from build123d import *

# Parameters (mm, degrees)
F0_W           = 127
F0_H           = 45.593
F1_DEPTH       = 19.05
F3_D           = 13.5128
F3_DEPTH       = 19.05
F3_CBORE_D     = 20.066
F3_CBORE_DEPTH = 13.4874
F3_TIP         = 4.0596546864
F5_DEPTH       = 45.593
F7_DEPTH       = 10.1854
F9_DEPTH       = 7.9375
F10_R          = 4.7625
F11_DEPTH      = 69.85
F12_R          = 4.76249
F4_R           = 4.7625


# Not quite as in the source:
# - a fillet or chamfer is up to 0.001 mm smaller than in the source, because OpenCascade refuses the exact size


with BuildPart() as f1:
    # F0 (on Front) → F1 (new body)
    with BuildSketch(Plane.XZ):
        with Locations((63.5, -22.7965)):
            Rectangle(F0_W, F0_H)
    extrude(amount=-F1_DEPTH)

    # F3
    with Locations(Plane.XZ):
        with Locations((14.3002, -21.7424), (112.7125, -21.7424)):
            CounterBoreHole(F3_D / 2, F3_CBORE_D / 2, F3_CBORE_DEPTH, depth=F3_DEPTH)
            with Locations((0, 0, -(F3_DEPTH + F3_TIP / 2))):  # 118° drill point
                Cone(0, F3_D / 2, F3_TIP, mode=Mode.SUBTRACT)

    # F4 (on face) → F5 (cut)
    with BuildSketch(Plane.XY):
        with BuildLine():
            Line((58.7375, 0), (68.2625, 0))
            ThreePointArc((68.2625, 0), (63.5, 4.7625), (58.7375, 0))
        make_face()
        with BuildLine():
            ThreePointArc((58.7375, 0), (63.5, -4.7625), (68.2625, 0))
            Line((68.2625, 0), (58.7375, 0))
        make_face()
    extrude(amount=-F5_DEPTH, mode=Mode.SUBTRACT)

    # F6 (on face) → F7 (cut)
    with BuildSketch(Plane.XZ):
        with BuildLine():
            Line((93.6498, 0), (76.2, 0))
            Line((76.2, 0), (76.2, -30.1625))
            ThreePointArc((76.2, -30.1625), (77.1299359697, -32.4075640303), (79.375, -33.3375))
            Line((79.375, -33.3375), (90.4748, -33.3375))
            ThreePointArc((90.4748, -33.3375), (92.7198640303, -32.4075640303), (93.6498, -30.1625))
            Line((93.6498, -30.1625), (93.6498, 0))
        make_face()
    extrude(amount=-F7_DEPTH, mode=Mode.SUBTRACT)

    # F8 (on Front) → F9 (cut)
    with BuildSketch(Plane.XZ):
        with BuildLine():
            Line((103.8733, 0), (95.9358, 0))
            Line((95.9358, 0), (95.9358, -22.1996))
            ThreePointArc((95.9358, -22.1996), (97.0963600902, -25.0014399098), (99.8982, -26.162))
            Line((99.8982, -26.162), (99.9109, -26.162))
            ThreePointArc((99.9109, -26.162), (102.7127399098, -25.0014399098), (103.8733, -22.1996))
            Line((103.8733, -22.1996), (103.8733, 0))
        make_face()
    extrude(amount=-F9_DEPTH, mode=Mode.SUBTRACT)

    # F10 (on face) → F11 (cut)
    with BuildSketch(Plane.YZ.offset(95.9358)):
        with Locations((0, -13.2588)):
            Circle(F10_R)
    extrude(amount=-F11_DEPTH, mode=Mode.SUBTRACT)

    # F12 (radius 4.7625 in the source; OpenCascade refuses exactly that, so slightly less here)
    f12_edges = [f1.edges().sort_by_distance(p)[0] for p in [
        (26.0858, 4.7625, -13.2588),
    ]]
    fillet(f12_edges, radius=F12_R)

    # F14: sweep along a path in F13
    with BuildLine(Plane.XZ) as f14_path:
        Line((63.5, 0), (63.5, -2.4638))
        ThreePointArc((63.5, -2.4638), (66.6617822971, -10.0970177029), (74.295, -13.2588))
        Line((74.295, -13.2588), (77.6987022404, -13.2588))
    # F4 (on face) → F14 (sweep, cut)
    with BuildSketch(Plane.XY):
        with Locations((63.5, 0)):
            Circle(F4_R)
    sweep(path=f14_path.line, mode=Mode.SUBTRACT)


solid = f1.part
Geometry: final body of the model. Coordinates: model frame, mm. A direction names the side the tool comes from. Give positions to 0.01 mm unless a question says otherwise; leave off trailing zeros. Write each loop counter-clockwise with the first axis right and the second up, starting at its lowest first coordinate (ties: lowest second). Pieces come first, ordered by that corner, then holes.
(1) Cut plane C-C, the plane y = 16.25. Return loops of the section in (x, z).
(2) Access query for faces 4 (the flat face through (95, 0, -4)), 5 (the flat face through (95.936, 5, -11)), 6 (the cylindrical face through (71.35, 4.438, -14.986)). Directions: +Z, -Z, +X, -X, +Y, -Y. A direction counts if a zero-diameter tool reaches every point of the face in a straight line with its end or side. Return the directions, or none.
(3) Cut plane A-A, the plane x = 80.5. Return loops of the section in (y, z).
(4) Mould query, pull axis Z, two halves, no side actions, for faces 1 (the flat face through (110.3, 13.487, -28.3)), 2 (the flat face through (103.873, 4, -9)), 3 (the cylindrical face through (97.066, 3.913, -24.97)). Classes: released by +Z, released by -Z, zero draft, split by the parting line, or undercut.
(5) Ray query, line 1 (X direction, y = 1.25, z = -5); line 2 (X direction, y = 8, z = -17); line 3 (Z direction, x = 80, y = 9.75). Return the intervals inside material, ascending.
(6) First-contact query: P1, Ø5, axis at x = 85.5, z = -12.5, coming from the -Y side; P2, Ø15.5, axis at x = 14.3, z = -21.74, coming from the -Y side; P3, Ø6.5, axis at x = 100, z = -11, coming from the -Y side. Flat tips, straight axial feed; report the tip coordinate or a pass-through.
(7) Cut plane B-B, the plane x = 113. Return loops of the section in (y, z), then the cut area to 3 significant figures.
Values follow:
1. outline: (0, -45.59) - (127, -45.59) - (127, 0) - (0, 0) - close; hole circle Ø13.51 at (14.3, -21.74); hole circle Ø13.51 at (112.71, -21.74)
2. face 4: +Z, -Z, +X, -X, -Y
2. face 5: +Z, -Y
2. face 6: -Y
3. outline: (0, -45.59) - (19.05, -45.59) - (19.05, 0) - (10.19, 0) - (10.19, -33.34) - (0, -33.34) - close
4. face 1: undercut
4. face 2: zero draft
4. face 3: released by +Z
5. line 1: x = 0 to 58.9, 68.64 to 76.2, 93.65 to 95.94, 103.87 to 127
5. line 2: x = 0 to 5.46, 23.14 to 76.2, 93.65 to 103.87, 121.55 to 127
5. line 3: z = -45.59 to -33.34
6. P1: stops at y = 10.19
6. P2: stops at y = 13.49
6. P3: stops at y = 7.94
7. outline: (0, -45.59) - (19.05, -45.59) - (19.05, -28.49) - (13.49, -28.49) - (13.49, -31.77) - (0, -31.77) - close; (0, -11.71) - (13.49, -11.71) - (13.49, -14.99) - (19.05, -14.99) - (19.05, 0) - (0, 0) - close
7. area: 523 mm2
